Can you work these out from the drawing? Everything is in mm from the part's minimum corner. A direction names the side the tool comes from. Coordinates: 2 decimals unless noted, no trailing zeros. Loops run counter-clockwise (first coordinate to the right, second up) from the corner with the lowest first, then second, coordinate; pieces in that order, holes last. Notation, with made-up numbers: (-4, 2.5) -> (10, 2.5) arc R27 cw to (10, 34.5) -> close; hole circle Ø8 at (46, 81). An arc over 180 degrees is marked (long way). Use one line per item in the form item = value. Start each with the question number.
(1) Thinking about a two-plate mould opening in Z: for the marked faces 1, 2 and 3, which applies, released by +Z, released by -Z, zero draft, split by the parting line, or undercut?
(2) Imagine slicing it at D-D (y = 5.5). List the corners of the cut face in (x, z) for me.
(3) Imagine slicing it at A-A (x = 0.8). List the corners of the cut face in (y, z) for me (1 decimal).
(4) Imagine slicing it at C-C (z = 5.75). List the corners of the cut face in (x, y) for me (1 decimal).
(5) Imagine slicing it at B-B (y = 14.5). List the corners of the cut face in (x, z) for me.
(6) On a 3-axis mill with a long thin cutter (end or side, diameter ignored), from which of +Z, -Z, +X, -X, +Y, -Y can I reach the whole of each face in a straight line? I mean the marked faces 4, 5, 6, 7 and 8. Say none if no direction works.
(7) I'm going to push flat-ended pins straight in: pin 1 (0.5 mm diameter, centred on x = 1, y = 5.5, fed in from +Z); pin 2 (0.9 mm diameter, centred on x = 1, y = 11.5, fed in from -Z); pin 3 (0.5 mm diameter, centred on x = 0.5, y = 12.5, fed in from +Z). Where does each tip first touch, or does it pass through?
(8) I need wall thicknesses on line 1 (Z direction, x = 0.3, y = 15.75); line 2 (Z direction, x = 1.1, y = 5.5) (1 decimal); line 3 (Z direction, x = 1.35, y = 17). Which ranges of each line are inside material? Lowest first, please. Write a range as [from, to].
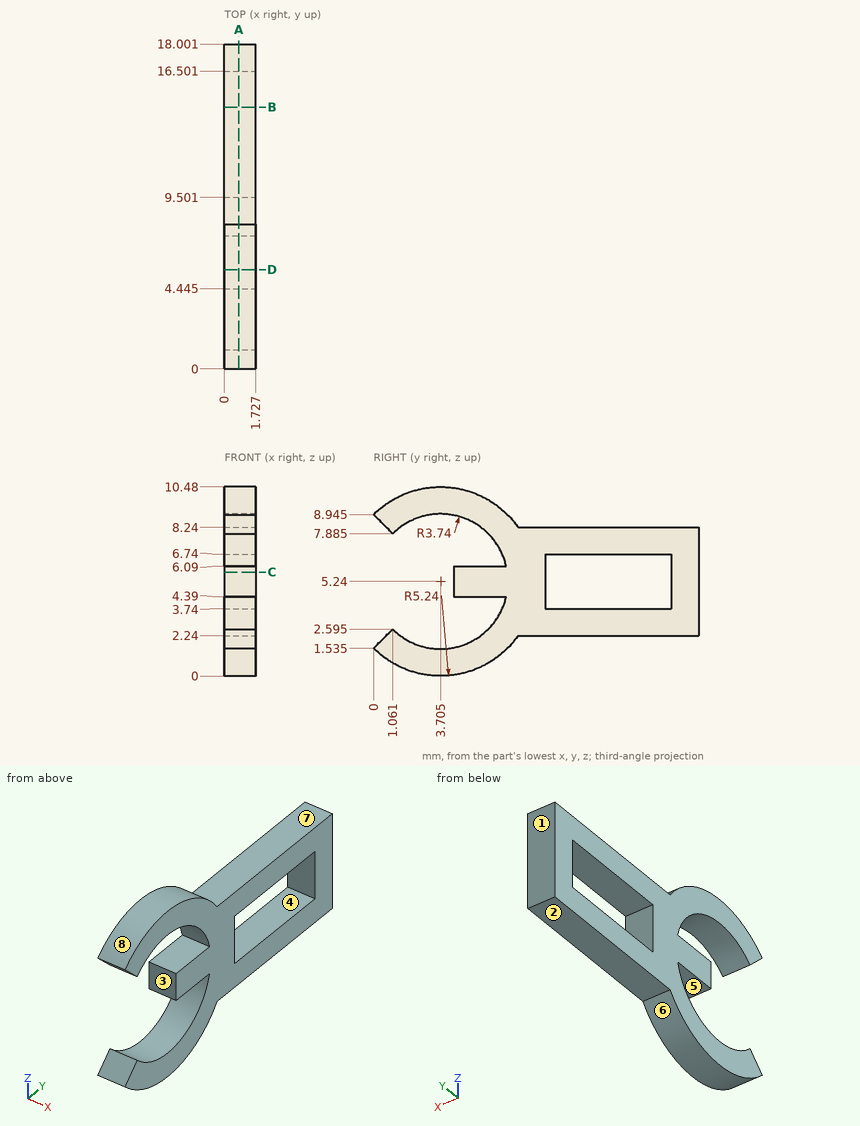
Worked out:
q1.face_1 = zero draft
q1.face_2 = released by -Z
q1.face_3 = undercut
q2.outline = (0, 0.32) -> (1.73, 0.32) -> (1.73, 1.96) -> (0, 1.96) -> close; (0, 4.39) -> (1.73, 4.39) -> (1.73, 6.09) -> (0, 6.09) -> close; (0, 8.52) -> (1.73, 8.52) -> (1.73, 10.16) -> (0, 10.16) -> close
q3.outline = (0, 1.5) arc R5.2 ccw to (8, 2.2) -> (18, 2.2) -> (18, 8.2) -> (8, 8.2) arc R5.2 ccw to (0, 8.9) -> (1.1, 7.9) arc R3.7 cw to (7.3, 6.1) -> (4.4, 6.1) -> (4.4, 4.4) -> (7.3, 4.4) arc R3.7 cw to (1.1, 2.6) -> close; hole (9.5, 3.7) -> (16.5, 3.7) -> (16.5, 6.7) -> (9.5, 6.7) -> close
q4.outline = (0, 4.4) -> (1.7, 4.4) -> (1.7, 9.5) -> (0, 9.5) -> close; (0, 16.5) -> (1.7, 16.5) -> (1.7, 18) -> (0, 18) -> close
q5.outline = (0, 2.24) -> (1.73, 2.24) -> (1.73, 3.74) -> (0, 3.74) -> close; (0, 6.74) -> (1.73, 6.74) -> (1.73, 8.24) -> (0, 8.24) -> close
q6.face_4 = +X, -X
q6.face_5 = +X, -X, -Y
q6.face_6 = -Z, +X, -X
q6.face_7 = +Z, +X, -X, +Y
q6.face_8 = +Z, +X, -X
q7.pin_1 = 10.25
q7.pin_2 = 2.24
q7.pin_3 = 8.24
q8.line_1 = [2.24, 3.74], [6.74, 8.24]
q8.line_2 = [0.3, 2], [4.4, 6.1], [8.5, 10.2]
q8.line_3 = [2.24, 8.24]
